Could you check a few things on this model? Use its own coordinates, in mm. A direction names the side the tool comes from. Give positions to 0.01 mm unless a question says otherwise; leave off trailing zeros. Loops run counter-clockwise (first coordinate to the right, second up) from the corner with the lowest first, then second, coordinate; pieces in that order, holes last. Notation, with made-up numbers: (80.5, -10.5) - (129.5, -10.5) arc R18 ccw to (129.5, 19.5) - close; hole circle Ø7 at (21, 10.25). An arc over 180 degrees is marked (long way). One line per item, written item: value. Start each with the question number.
Q1. I'm going to push flat-ended pins straight in: P1, Ø3, axis at x = -102, y = 15, coming from the +Z side; P2, Ø13, axis at x = -126.5, z = 26.5, coming from the +Y side; P3, Ø7.5, axis at x = -127, z = 25.4, coming from the -Y side; P4, Ø12, axis at x = -116, y = 24, coming from the -Z side. Where does each tip first touch, or does it pass through?
Q2. I want a section at A-A (z = -25.4). Please give me the cut outline in (x, y) (3 decimals), then the cut area to 3 significant figures.
Q3. For faces 1 (the face through (-127.41, 2.46, 22.25)), 2 (the face through (-131.42, 7.03, 21.34)), 3 (the face through (-129.692, 4.93, -7.339)), which set-ups out of +Z, -Z, +X, -X, +Y, -Y let a thin tool reach every point of the face, with its end or its side?
Q4. I want a section at C-C (x = -100). Please give me the cut outline in (y, z), then the cut area to 3 significant figures.
Q5. I want a section at D-D (x = -118). Please give me the cut outline in (y, z).
Q6. I want a section at B-B (y = 15.25). Please give me the cut outline in (x, z).
Q7. If I drill on line 1 (X direction, y = 8.5, z = 0); line 2 (Z direction, x = -127, y = 7.55); line 3 (Z direction, x = -127, y = 3.8) (3 decimals), over which ranges is the centre line in solid material (lowest first)? Write a range as from..to.
Q8. If we mould it in two halves opening along X, with no side actions, what happens to faces 4 (the face through (-129.48, 4.93, 7.14)), 5 (the face through (-103.033, 4.93, -23.448)), 6 (the face through (-124, 5, -23)), 7 (the face through (-137.697, 4.93, -35.916))? For each: released by +X, released by -X, zero draft, split by the parting line, or undercut.
```python
from build123d import *

# Parameters (mm, degrees)
SKETCH4_R           = 3.175
BOSS_EXTRUDE1_DEPTH = 10
SKETCH5_R           = 15
BOSS_EXTRUDE2_DEPTH = 20
SKETCH6_R           = 2.85
CUT_EXTRUDE1_DEPTH  = 38
SKETCH7_R           = 6
CUT_EXTRUDE2_DEPTH  = 5
SKETCH8_R           = 6
CUT_EXTRUDE3_DEPTH  = 5
CHAMFER1_SIZE       = 1


with BuildPart() as part:
    # Sketch4 → Boss-Extrude1 (new body)
    with BuildSketch(Plane(origin=(0, 0, 0), x_dir=(1, 0, 0), z_dir=(0, 1, 0))):
        with BuildLine():
            Line((-89.722054171, 10.925375487), (-116.722054171, 36.325375487))
            ThreePointArc((-116.722054171, 36.325375487), (-137.925375487, 35.677945829), (-137.277945829, 14.474624513))
            Line((-137.277945829, 14.474624513), (-121.891533945, 0))
            Line((-121.891533945, 0), (-137.277945829, -14.474624513))
            ThreePointArc((-137.277945829, -14.474624513), (-137.925375487, -35.677945829), (-116.722054171, -36.325375487))
            Line((-116.722054171, -36.325375487), (-89.722054171, -10.925375487))
            ThreePointArc((-89.722054171, -10.925375487), (-85, 0), (-89.722054171, 10.925375487))
        make_face()
        with Locations((-127, 25.4)):
            Circle(SKETCH4_R, mode=Mode.SUBTRACT)
        with Locations((-127, -25.4)):
            Circle(SKETCH4_R, mode=Mode.SUBTRACT)
    extrude(amount=BOSS_EXTRUDE1_DEPTH)

    # Sketch5 → Boss-Extrude2 (add)
    with BuildSketch(Plane(origin=(0, 10, 0), x_dir=(1, 0, 0), z_dir=(0, 1, 0))):
        with Locations((-100, 0)):
            Circle(SKETCH5_R)
    extrude(amount=BOSS_EXTRUDE2_DEPTH)

    # Sketch6 → Cut-Extrude1 (cut)
    with BuildSketch(Plane(origin=(0, 30, 0), x_dir=(1, 0, 0), z_dir=(0, 1, 0))):
        with Locations((-100, 0)):
            Circle(SKETCH6_R)
    extrude(amount=-CUT_EXTRUDE1_DEPTH, mode=Mode.SUBTRACT)

    # Sketch7 → Cut-Extrude2 (cut)
    with BuildSketch(Plane(origin=(0, 10, 0), x_dir=(1, 0, 0), z_dir=(0, 1, 0))):
        with Locations((-127, -25.4)):
            Circle(SKETCH7_R)
    extrude(amount=-CUT_EXTRUDE2_DEPTH, mode=Mode.SUBTRACT)

    # Sketch8 → Cut-Extrude3 (cut)
    with BuildSketch(Plane(origin=(0, 10, 0), x_dir=(1, 0, 0), z_dir=(0, 1, 0))):
        with Locations((-127, 25.4)):
            Circle(SKETCH8_R)
    extrude(amount=-CUT_EXTRUDE3_DEPTH, mode=Mode.SUBTRACT)

    # Chamfer1
    chamfer1_edges = [part.edges().sort_by_distance(p)[0] for p in [
        (-102.85, 30, 0),
        (-133, 10, 25.4),
        (-133, 10, -25.4),
    ]]
    chamfer(chamfer1_edges, length=CHAMFER1_SIZE)


solid = part.part
```
Worked answers:
1. P1: stops at z = 14.99
1. P2: stops at y = 10
1. P3: stops at y = 0
1. P4: stops at z = -11.18
2. outline: (-142, 0) - (-130.175, 0) - (-130.175, 5) - (-133, 5) - (-133, 9) - (-134, 10) - (-142, 10) - close; (-123.825, 0) - (-105.108, 0) - (-105.108, 10) - (-120, 10) - (-121, 9) - (-121, 5) - (-123.825, 5) - close
2. area: 276 mm²
3. face 1: +Y, -Y
3. face 2: +Y
3. face 3: -X, +Y, -Y
4. outline: (0, -20.59) - (10, -20.59) - (10, -15) - (30, -15) - (30, -3.85) - (29, -2.85) - (0, -2.85) - close; (0, 2.85) - (29, 2.85) - (30, 3.85) - (30, 15) - (10, 15) - (10, 20.59) - (0, 20.59) - close
4. area: 840 mm²
5. outline: (0, -37.4) - (10, -37.4) - (10, 37.4) - (0, 37.4) - close
6. outline: circle Ø30 at (-100, 0); hole circle Ø5.7 at (-100, 0)
7. line 1: x = -121.89..-102.85, -97.15..-85
7. line 2: z = -40.4..-31.4, -19.4..-4.81, 4.81..19.4, 31.4..40.4
7. line 3: z = -40.4..-28.575, -22.225..-4.806, 4.806..22.225, 28.575..40.4
8. face 4: released by -X
8. face 5: released by +X
8. face 6: undercut
8. face 7: split by the parting line
